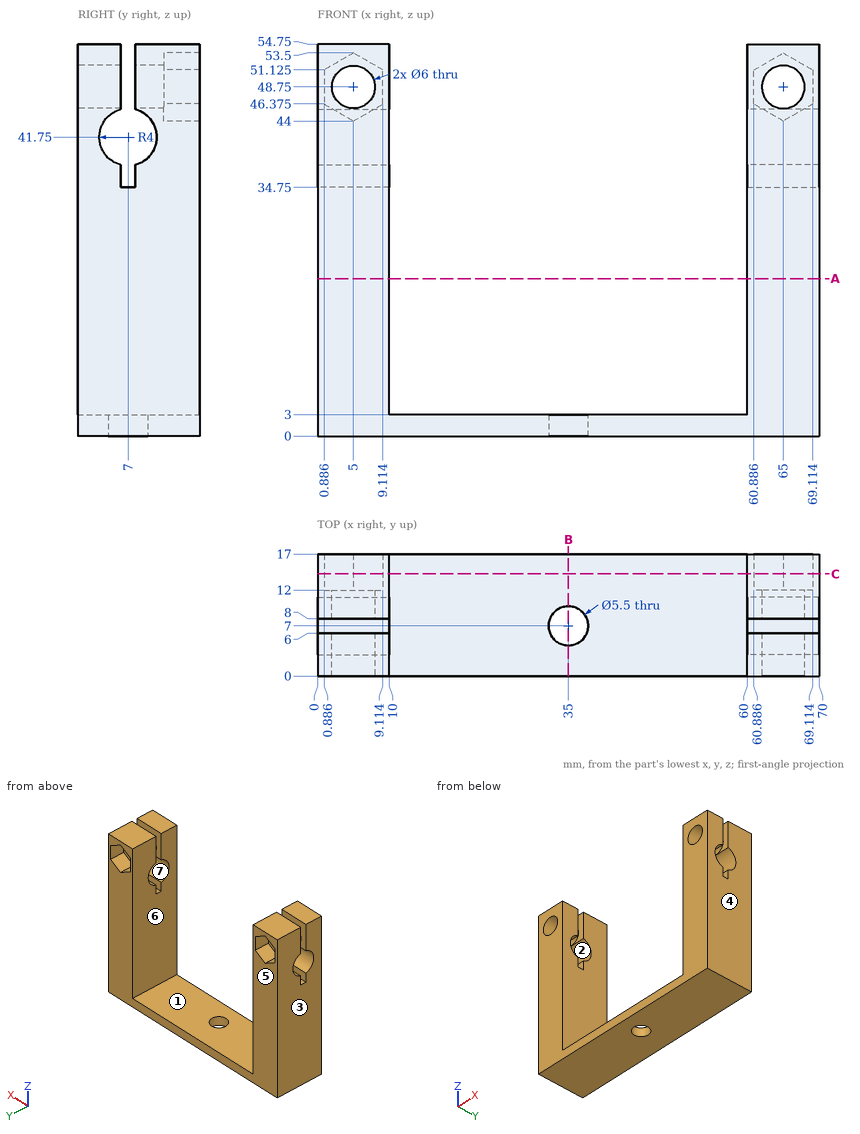
Answer from the drawing. Dimensions are ordinates in mm from the lowest x, y and z of the part. A direction names the side the tool comes from. Coordinates: 2 decimals unless noted, no trailing zeros. Loops run counter-clockwise (first coordinate to the right, second up) from the corner with the lowest first, then second, coordinate; pieces in that order, holes last. Notation, with made-up numbers: (29.25, 10) -> (88.25, 10) arc R21 cw to (88.25, 20) -> close; hole circle Ø8 at (35.5, -24). An arc over 180 degrees is marked (long way). Answer as CSV lines item,"result".
Q1. Each of these flat-tipped pins is pushed along its axis until it touches: pin 1 (5.5 mm diameter, centred on x = 5, z = 48.75, fed in from -Y); pin 2 (6 mm diameter, centred on x = 42, y = 9, fed in from +Z). Where does it stop, or does it pass through?
Findings:
pin 1,"passes through"
pin 2,"stops at z = 3"
Q2. The part is cut by section A-A on z = 22. Write down the section's boundary in (x, y), and give its area (3 significant figures).
Findings:
outline,"(0, 0) -> (10, 0) -> (10, 17) -> (0, 17) -> close; (60, 0) -> (70, 0) -> (70, 17) -> (60, 17) -> close"
area,"340 mm²"
Q3. The part is cut by section C-C on y = 14.25. State how many separate pieces and enclosed holes the cut face has, and give its area (3 significant figures).
Findings:
separate pieces,"1"
enclosed holes,"2"
area,"1,130 mm²"
Q4. The part is cut by section B-B on x = 35. Write down the section's boundary in (y, z), and give its area (3 significant figures).
Findings:
outline,"(0, 0) -> (4.25, 0) -> (4.25, 3) -> (0, 3) -> close; (9.75, 0) -> (17, 0) -> (17, 3) -> (9.75, 3) -> close"
area,"34.5 mm²"
Q5. For a pull along X with two mould halves and no side action, classify the marked faces 1, 2, 3 and 4 as +X half, -X half, draft (parallel to the pull), parting line (faces both ways), or undercut.
Findings:
face 1,"undercut"
face 2,"draft"
face 3,"-X half"
face 4,"+X half"
Q6. A tool of negligible diameter and unlimited length cuts with its end or side. For the marked faces 5, 6 and 7, from which of +Z, -Z, +X, -X, +Y, -Y can it reach the whole face along a straight path? Write none if from no direction.
Findings:
face 5,"+Z, -Z, +X, -X, +Y"
face 6,"+Z, +Y, -Y"
face 7,"+X, -X"
Q7. Find the intervals of material crossed by probe 1 along X at (y, z) = (16, 50.5); probe 2 along X at (y, z) = (2.75, 6); probe 3 along X at (y, z) = (7, 0.9), in increasing order.
Findings:
probe 1,"x = 0 to 0.89, 9.11 to 10, 60 to 60.89, 69.11 to 70"
probe 2,"x = 0 to 10, 60 to 70"
probe 3,"x = 0 to 32.25, 37.75 to 70"
